Verification items for the finished model (mm, model axes). A direction names the side the tool comes from. Coordinates: 2 decimals unless noted, no trailing zeros. Write each loop counter-clockwise with the first axis right and the second up, starting at its lowest first coordinate (ties: lowest second). Pieces come first, ordered by that corner, then holes. Notation, with made-up numbers: (54, 21) -> (73, 21) arc R26 cw to (73, 58) -> close; hole circle Ø9 at (67, 3). An arc over 180 degrees is marked (long way). Answer in a Markdown table with one row per item.
```python
from build123d import *

# Parameters (mm, degrees)
FILLET1_R           = 0.25
BOSS_EXTRUDE1_DEPTH = 3
FILLET2_R           = 3


with BuildPart() as part:
    # BodySke → Base-Revolve (revolve)
    with BuildSketch(Plane.XY):
        Polygon((0, 0), (0, 3), (15.4455, 3), (16, 2.4455), (16, 0), align=None)
    revolve(axis=Axis((-31.75, 0, 0), (1, 0, 0)))

    # Fillet1
    fillet1_edges = [part.edges().sort_by_distance(p)[0] for p in [
        (0, -3, 0),
    ]]
    fillet(fillet1_edges, radius=FILLET1_R)

    # Sketch1 → Boss-Extrude1 (add, symmetric)
    with BuildSketch(Plane.XY):
        Polygon((-5.5, -3.4), (-5.5, 3.4), (-2.9, 6), (-1.5, 6), (-1.5, 3), (0, 3), (0, -3), (-1.5, -3), (-1.5, -6), (-2.9, -6), align=None)
    extrude(amount=BOSS_EXTRUDE1_DEPTH, both=True)

    # Fillet2
    fillet2_edges = [part.edges().sort_by_distance(p)[0] for p in [
        (-0.75, 3, -3),
        (-0.75, -3, 3),
    ]]
    fillet(fillet2_edges, radius=FILLET2_R)


solid = part.part
```
1. Tool access check on faces 1 (the cylindrical face through (8, -3, 0)), 2 (the flat face through (-1, -3, -1)), 3 (the cylindrical face through (-0.74, 2.1, -2.14)), 4 (the cylindrical face through (-0.76, -2.1, 2.14)). Record the directions out of +Z, -Z, +X, -X, +Y, -Y that give a thin tool (end or side, any length) a straight path to the whole face; none if there is none.
Geometry says:
| item | result |
|---|---|
| face 1 | +X |
| face 2 | +Z, -Z, +X, -Y |
| face 3 | -Z, +X, +Y |
| face 4 | +Z, +X, -Y |
2. Thickness scan on line 1 (X direction, y = 3.25, z = -1.5); line 2 (X direction, y = -4, z = 2.25); line 3 (Y direction, x = 2.75, z = 1.5). Record the ranges inside material, lowest first. Write a range as from..to.
Geometry says:
| item | result |
|---|---|
| line 1 | -5.5..-1.5 |
| line 2 | -4.9..-1.5 |
| line 3 | -2.6..2.6 |
3. Depth check by flat-ended pin: P1, Ø3, axis at y = -3, z = -0.5, coming from the +X side; P2, Ø0.8, axis at x = -1, z = -1.5, coming from the -Y side; P3, Ø4, axis at x = 8.5, y = 4.5, coming from the -Z side. Enter the tip coordinate at first touch or a pass-through.
Geometry says:
| item | result |
|---|---|
| P1 | x = 16 |
| P2 | y = -3 |
| P3 | z = -1.66 |
4. Section check A-A, the plane x = 3. Record the boundary of the cut face in (y, z).
Geometry says:
| item | result |
|---|---|
| outline | circle Ø6 at (0, 0) |
5. Section check B-B, the plane y = -4.25. Record the boundary of the cut face in (x, z).
Geometry says:
| item | result |
|---|---|
| outline | (-4.65, -3) -> (-1.5, -3) -> (-1.5, 3) -> (-4.65, 3) -> close |
